Job drawing, mm, ordinate dimensions from the low corner. One solid piece. A direction names the side the tool comes from. Give positions to 0.01 mm unless a question says otherwise; leave off trailing zeros. Order: outer loops, then holes, each group sorted by start corner. A loop starts at its lowest first (then second) coordinate and runs counter-clockwise, first axis right, second up. Notation, with made-up numbers: (74.25, 54) - (127.25, 54) arc R31 cw to (127.25, 81) - close; hole circle Ø5 at (80.25, 88.25). An arc over 180 degrees is marked (long way). One line per item, written item: value.
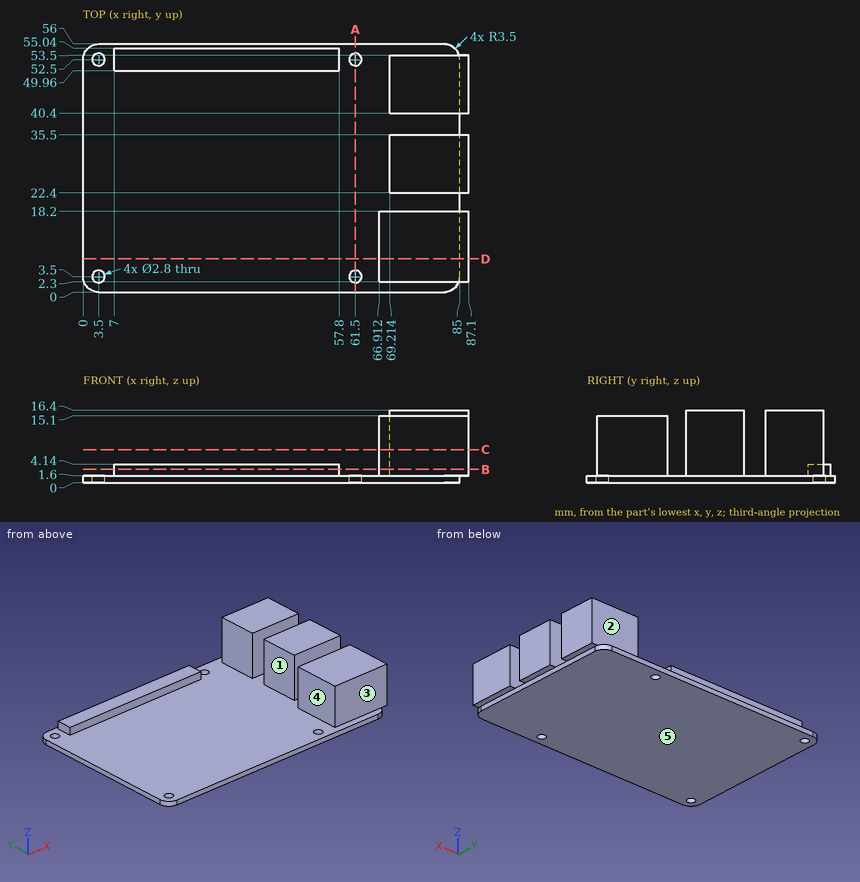
1) Slice it at D-D on y = 7.5. Write the cut outline in (x, z).
Answer:
outline: (0, 0) - (85, 0) - (85, 1.6) - (87.1, 1.6) - (87.1, 15.1) - (66.91, 15.1) - (66.91, 1.6) - (0, 1.6) - close
2) Wall check: line 1 along Y through (x, z) = (61.5, 0.7); line 2 along X through (y, z) = (52.5, 0.5); line 3 along Y through (x, z) = (77, 15.75). Give the ranges that are in metal, low to high. Write a range as [from, to].
Answer:
line 1: y = [0, 2.1], [4.9, 51.1], [53.9, 56]
line 2: x = [0, 2.1], [4.9, 60.1], [62.9, 85]
line 3: y = [22.4, 35.5], [40.4, 53.5]
3) Slice it at C-C on z = 7.5. Write the cut outline in (x, y).
Answer:
outline: (66.91, 2.3) - (87.1, 2.3) - (87.1, 18.2) - (66.91, 18.2) - close; (69.21, 22.4) - (87.1, 22.4) - (87.1, 35.5) - (69.21, 35.5) - close; (69.21, 40.4) - (87.1, 40.4) - (87.1, 53.5) - (69.21, 53.5) - close
4) Which spindle directions (+Z, -Z, +X, -X, +Y, -Y) get a long thin tool onto all of the face, cutting with end or side? Do the marked faces 1, 2, 3, 4 and 5. Say none if no direction does.
Answer:
face 1: +Z, -X, +Y
face 2: +Z, +X, +Y
face 3: +Z, +X, -X, -Y
face 4: +Z, -X, +Y, -Y
face 5: -Z, +X, -X, +Y, -Y
5) Slice it at A-A on x = 61.5. Write the cut outline in (y, z).
Answer:
outline: (0, 0) - (2.1, 0) - (2.1, 1.6) - (0, 1.6) - close; (4.9, 0) - (51.1, 0) - (51.1, 1.6) - (4.9, 1.6) - close; (53.9, 0) - (56, 0) - (56, 1.6) - (53.9, 1.6) - close
6) Slice it at B-B on z = 3. Write the cut outline in (x, y), then the cut area to 3 significant figures.
Answer:
outline: (7, 49.96) - (57.8, 49.96) - (57.8, 55.04) - (7, 55.04) - close; (66.91, 2.3) - (87.1, 2.3) - (87.1, 18.2) - (66.91, 18.2) - close; (69.21, 22.4) - (87.1, 22.4) - (87.1, 35.5) - (69.21, 35.5) - close; (69.21, 40.4) - (87.1, 40.4) - (87.1, 53.5) - (69.21, 53.5) - close
area: 1,050 mm2
7) Drop flat-ended pins along their axis: P1, Ø5, axis at x = 77, y = 10.5, coming from the +Z side; P2, Ø3.5, axis at x = 3.5, y = 3.5, coming from the +Z side; P3, Ø7.5, axis at x = 80.5, z = 12.5, coming from the +Y side; P4, Ø2, axis at x = 3.5, y = 52.5, coming from the +Z side. Give the stop position or say it passes through.
Answer:
P1: stops at z = 15.1
P2: stops at z = 1.6
P3: stops at y = 53.5
P4: passes through
